from build123d import *

# Parameters (mm, degrees)
PAD_DEPTH       = 2
SKETCH002_R     = 1.5
POCKET_DEPTH    = 5
CHAMFER_SIZE    = 1
CHAMFER001_SIZE = 1
CHAMFER002_SIZE = 1
CHAMFER003_SIZE = 1
SKETCH004_W     = 50
SKETCH004_H     = 30
POCKET001_DEPTH = 5
PAD001_DEPTH    = 2


with BuildPart() as part:
    # Sketch → Pad (new body)
    with BuildSketch(Plane.XY):
        with BuildLine():
            Line((-64.5, 49.5), (64.5, 49.5))
            ThreePointArc((74.5, 39.5), (71.571068, 46.571068), (64.5, 49.5))
            Line((74.5, 39.5), (74.5, -39.5))
            ThreePointArc((64.5, -49.5), (71.571068, -46.571068), (74.5, -39.5))
            Line((64.5, -49.5), (-64.5, -49.5))
            ThreePointArc((-74.5, -39.5), (-71.571068, -46.571068), (-64.5, -49.5))
            Line((-74.5, -39.5), (-74.5, 39.5))
            ThreePointArc((-64.5, 49.5), (-71.571068, 46.571068), (-74.5, 39.5))
        make_face()
    extrude(amount=PAD_DEPTH)

    # Sketch002 → Pocket (cut)
    with BuildSketch(Plane.XY.offset(4)):
        with Locations((-68, 43)):
            Circle(SKETCH002_R)
        with Locations((-68, -43)):
            Circle(SKETCH002_R)
        with Locations((68, -43)):
            Circle(SKETCH002_R)
        with Locations((68, 43)):
            Circle(SKETCH002_R)
    extrude(amount=-POCKET_DEPTH, mode=Mode.SUBTRACT)

    # Chamfer
    chamfer_edges = [part.edges().sort_by_distance(p)[0] for p in [
        (-69.5, 43, 0),
    ]]
    chamfer(chamfer_edges, length=CHAMFER_SIZE)

    # Chamfer001
    chamfer001_edges = [part.edges().sort_by_distance(p)[0] for p in [
        (-69.5, -43, 0),
    ]]
    chamfer(chamfer001_edges, length=CHAMFER001_SIZE)

    # Chamfer002
    chamfer002_edges = [part.edges().sort_by_distance(p)[0] for p in [
        (66.5, -43, 0),
    ]]
    chamfer(chamfer002_edges, length=CHAMFER002_SIZE)

    # Chamfer003
    chamfer003_edges = [part.edges().sort_by_distance(p)[0] for p in [
        (66.5, 43, 0),
    ]]
    chamfer(chamfer003_edges, length=CHAMFER003_SIZE)

    # Sketch004 → Pocket001 (cut)
    with BuildSketch(Plane(origin=(0, 0, 0), x_dir=(1, 0, 0), z_dir=(0, 0, -1))):
        Rectangle(SKETCH004_W, SKETCH004_H)
    extrude(amount=-POCKET001_DEPTH, mode=Mode.SUBTRACT)

    # Sketch005 (on Face18 of Pocket001) → Pad001 (join)
    with BuildSketch(Plane.XY.offset(2)):
        Polygon((-57, 47), (57, 47), (72, 32), (72, -32), (57, -47), (-57, -47), (-72, -32), (-72, 32), align=None)
        Polygon((-70.5, 31.25), (-56.25, 45.5), (56.25, 45.5), (70.5, 31.25), (70.5, -31.25), (56.25, -45.5), (-56.25, -45.5), (-70.5, -31.25), align=None, mode=Mode.SUBTRACT)
    extrude(amount=PAD001_DEPTH)


solid = part.part
For this review, take the finished solid that the model builds, in its own axes (mm). A direction names the side the tool comes from. Round coordinates to 2 decimals unless told otherwise and drop trailing zeros. Loops run counter-clockwise (first coordinate to the right, second up) from the corner with the lowest first, then second, coordinate; pieces in that order, holes last. Notation, with made-up numbers: (7.5, -14) - (19.5, -14) arc R10 cw to (19.5, 2) - close; hole circle Ø8 at (49, 23). An arc over 180 degrees is marked (long way). Use one line per item in the form item = value.
Item 1: Consider section D-D on x = 68. Write out the cut boundary in (y, z).
Answers:
outline = (-48.87, 0) - (-45.5, 0) - (-44.5, 1) - (-44.5, 2) - (-48.87, 2) - close; (-41.5, 1) - (-40.5, 0) - (40.5, 0) - (41.5, 1) - (41.5, 2) - (36, 2) - (36, 4) - (33.75, 4) - (33.75, 2) - (-33.75, 2) - (-33.75, 4) - (-36, 4) - (-36, 2) - (-41.5, 2) - close; (44.5, 1) - (45.5, 0) - (48.87, 0) - (48.87, 2) - (44.5, 2) - close
Item 2: Consider section B-B on z = 2.9. Write out the cut boundary in (x, y).
Answers:
outline = (-72, -32) - (-57, -47) - (57, -47) - (72, -32) - (72, 32) - (57, 47) - (-57, 47) - (-72, 32) - close; hole (-70.5, -31.25) - (-56.25, -45.5) - (56.25, -45.5) - (70.5, -31.25) - (70.5, 31.25) - (56.25, 45.5) - (-56.25, 45.5) - (-70.5, 31.25) - close
Item 3: Clearance check with flat-ended pins moving along their axes: P1, Ø1, axis at x = -21, z = 3, coming from the +Y side; P2, Ø1, axis at x = 9.5, z = 3, coming from the -Y side; P3, Ø0.6, axis at y = 11.5, z = 3, coming from the -X side. State where each tip first meets the part, or that it passes through.
Answers:
P1 = 47
P2 = -47
P3 = -72
Item 4: Tool access review of faces 1 (the flat face through (65, -39, 3)), 2 (the flat face through (11.4, -47.4, 2)), 3 (the flat face through (-65, 39, 3)): name each direction out of +Z, -Z, +X, -X, +Y, -Y from which nothing blocks a thin tool from reaching the whole face with its end or side.
Answers:
face_1 = +Z, +X, -Y
face_2 = +Z
face_3 = +Z, -X, +Y
Item 5: For line 1 (X direction, y = -21.5, z = 3.45); line 2 (Y direction, x = 49.5, z = 2.85); line 3 (X direction, y = 5, z = 1.25), list the stretches that pass through material, from the lowest coordinate up.
Answers:
line_1 = -72 to -70.5, 70.5 to 72
line_2 = -47 to -45.5, 45.5 to 47
line_3 = -74.5 to -25, 25 to 74.5
Item 6: Consider section A-A on x = -10. Write out the cut boundary in (y, z), then the cut area to 3 significant figures.
Answers:
outline = (-49.5, 0) - (-15, 0) - (-15, 2) - (-45.5, 2) - (-45.5, 4) - (-47, 4) - (-47, 2) - (-49.5, 2) - close; (15, 0) - (49.5, 0) - (49.5, 2) - (47, 2) - (47, 4) - (45.5, 4) - (45.5, 2) - (15, 2) - close
area = 144 mm^2
Item 7: Consider section C-C on y = 2.5. Write out the cut boundary in (x, z), then the cut area to 3 significant figures.
Answers:
outline = (-74.5, 0) - (-25, 0) - (-25, 2) - (-70.5, 2) - (-70.5, 4) - (-72, 4) - (-72, 2) - (-74.5, 2) - close; (25, 0) - (74.5, 0) - (74.5, 2) - (72, 2) - (72, 4) - (70.5, 4) - (70.5, 2) - (25, 2) - close
area = 204 mm^2
Item 8: Mouldability with a two-part tool opening along Y and no side actions: class faces 4 (the flat face through (64, 40, 3)), 5 (the cylindrical face through (-67.31, -44.33, 1.51)), 6 (the flat face through (1, -20, 2)), 7 (the flat face through (-64, -40, 3)) as +Y half, -Y half, draft (parallel to the pull), parting line (faces both ways), or undercut.
Answers:
face_4 = +Y half
face_5 = undercut
face_6 = undercut
face_7 = -Y half
